For this review, take the finished solid that the model builds, in its own axes (mm). A direction names the side the tool comes from. Coordinates: 2 decimals unless noted, no trailing zeros. Write each loop counter-clockwise with the first axis right and the second up, starting at its lowest first coordinate (ties: lowest second). Pieces come first, ordered by that corner, then holes.
1) To check wall thickness, follow line 1 along Y through (x, z) = (85, 12.75); line 2 along Y through (x, z) = (70, 2.8); line 3 along X through (y, z) = (-21, 1.5). State the ranges of each line that lie inside material, in increasing order.
2) For faces 4 (the face through (68, 33.5, 10.6)), 5 (the face through (-87, 26, 6)), list the 3-axis set-ups (+Z, -Z, +X, -X, +Y, -Y) from which the entire face can be reached by the end or side of a thin tool; tool diameter is ignored.
3) We need section A-A on x = -89.5. Write out the cut boundary in (y, z), then the cut area to 3 significant figures.
4) We need section B-B on z = 2.5. Write out the cut boundary in (x, y), then the cut area to 3 significant figures.
5) Mouldability with a two-part tool opening along Y and no side actions: class faces 1 (the face through (67.5, -19.9, 10.6)), 2 (the face through (-1, -75, 7)), 3 (the face through (-100, -1, 7)) as pulls with the +Y half, pulls with the -Y half, needs draft (parallel to the pull), parting line crosses it, or undercut.
6) We need section C-C on y = 27.5. Write out the cut boundary in (x, z).
7) Insertion check: P1, Ø6.5, axis at x = 85, y = 20, coming from the -Z side. The pin has a flat end and moves straight along its axis. Give the tip position at first contact, or say it passes through.
from build123d import *

# Parameters (mm, degrees)
SKETCH1_W           = 200
SKETCH1_H           = 150
BOSS_EXTRUDE1_DEPTH = 15
SKETCH2_R           = 2.5
CUT_EXTRUDE1_DEPTH  = 126.89678312
SKETCH3_R           = 5
CUT_EXTRUDE2_DEPTH  = 6


with BuildPart() as part:
    # Sketch1 → Boss-Extrude1 (new body)
    with BuildSketch(Plane.XY):
        Rectangle(SKETCH1_W, SKETCH1_H)
    extrude(amount=BOSS_EXTRUDE1_DEPTH)

    # Sketch2 → Cut-Extrude1 (cut, through all)
    with BuildSketch(Plane.XY.offset(15)):
        with Locations((85, -35)):
            Circle(SKETCH2_R)
        with Locations((70, -20)):
            Circle(SKETCH2_R)
        with Locations((85, 20)):
            Circle(SKETCH2_R)
        with Locations((70, 35)):
            Circle(SKETCH2_R)
        with Locations((-89.5, 27.5)):
            Circle(SKETCH2_R)
        with Locations((-89.5, -27.5)):
            Circle(SKETCH2_R)
    extrude(amount=-CUT_EXTRUDE1_DEPTH, mode=Mode.SUBTRACT)

    # Sketch3 → Cut-Extrude2 (cut)
    with BuildSketch(Plane(origin=(0, 0, 0), x_dir=(-1, 0, 0), z_dir=(0, 0, -1))):
        with Locations((-70, 35)):
            Circle(SKETCH3_R)
        with Locations((-85, 20)):
            Circle(SKETCH3_R)
        with Locations((-70, -20)):
            Circle(SKETCH3_R)
        with Locations((-85, -35)):
            Circle(SKETCH3_R)
        with Locations((89.5, -27.5)):
            Circle(SKETCH3_R)
        with Locations((89.5, 27.5)):
            Circle(SKETCH3_R)
    extrude(amount=-CUT_EXTRUDE2_DEPTH, mode=Mode.SUBTRACT)


solid = part.part
Result:
1. line 1: y = -75 to -37.5, -32.5 to 17.5, 22.5 to 75
1. line 2: y = -75 to -25, -15 to 30, 40 to 75
1. line 3: x = -100 to 65.1, 74.9 to 100
2. face 4: +Z, -Z
2. face 5: -Z
3. outline: (-75, 0) - (-32.5, 0) - (-32.5, 6) - (-30, 6) - (-30, 15) - (-75, 15) - close; (-25, 6) - (-22.5, 6) - (-22.5, 0) - (22.5, 0) - (22.5, 6) - (25, 6) - (25, 15) - (-25, 15) - close; (30, 6) - (32.5, 6) - (32.5, 0) - (75, 0) - (75, 15) - (30, 15) - close
3. area: 2,040 mm2
4. outline: (-100, -75) - (100, -75) - (100, 75) - (-100, 75) - close; hole circle Ø10 at (-89.5, -27.5); hole circle Ø10 at (-89.5, 27.5); hole circle Ø10 at (70, -20); hole circle Ø10 at (70, 35); hole circle Ø10 at (85, -35); hole circle Ø10 at (85, 20)
4. area: 29,500 mm2
5. face 1: undercut
5. face 2: pulls with the -Y half
5. face 3: needs draft
6. outline: (-100, 0) - (-94.5, 0) - (-94.5, 6) - (-92, 6) - (-92, 15) - (-100, 15) - close; (-87, 6) - (-84.5, 6) - (-84.5, 0) - (100, 0) - (100, 15) - (-87, 15) - close
7. P1: stops at z = 6
